Here's how the part is built. I have some questions about the finished solid (model axes, mm). A direction names the side the tool comes from. Round coordinates to 2 decimals unless told otherwise and drop trailing zeros. Order: outer loops, then holes, each group sorted by start corner. A loop starts at its lowest first (then second) coordinate and runs counter-clockwise, first axis right, second up. Notation, with made-up numbers: (68, -35.75) -> (77, -35.75) arc R37 ccw to (77, 0.25) -> close; hole circle Ø9 at (52, 25.5). An arc over 180 degrees is marked (long way). Answer in a Markdown table with one row per item.
```python
from build123d import *

# Parameters (mm, degrees)
SKETCH2_W     = 0.9
SKETCH2_H     = 0.2
CHAMFER1_SIZE = 0.8
CHAMFER2_SIZE = 0.3


with BuildPart() as part:
    # Sketch1 → Revolve1 (revolve)
    with BuildSketch(Plane(origin=(0, 0, 0), x_dir=(0, 0, -1), z_dir=(1, 0, 0))):
        Polygon((-400, 0), (400, 0), (400, 4), (390, 4), (390, 6.32), (-346, 6.32), (-346, 4.94), (-385, 4.94), (-385, 4), (-400, 4), align=None)
    revolve(axis=Axis((0, 0, 400), (0, 0, -1)))

    # Sketch2 → Cut-Revolve1 (revolve, cut)
    with BuildSketch(Plane(origin=(0, 0, 0), x_dir=(0, 0, -1), z_dir=(1, 0, 0))):
        with Locations((397.45, 3.9)):
            Rectangle(SKETCH2_W, SKETCH2_H)
    revolve(axis=Axis((0, 0, -400), (0, 0, 1)), mode=Mode.SUBTRACT)

    # Chamfer1
    chamfer1_edges = [part.edges().sort_by_distance(p)[0] for p in [
        (0, -4, -400),
    ]]
    chamfer(chamfer1_edges, length=CHAMFER1_SIZE)

    # Chamfer2
    chamfer2_edges = [part.edges().sort_by_distance(p)[0] for p in [
        (0, -4.94, 385),
        (0, -4, 400),
    ]]
    chamfer(chamfer2_edges, length=CHAMFER2_SIZE)


solid = part.part
```
1. For faces 1 (the face through (-2, -5, 346)), 2 (the face through (-1.3, -4.1, -390)), 3 (the face through (5.329, 3.398, -16.848)), which set-ups out of +Z, -Z, +X, -X, +Y, -Y let a thin tool reach every point of the face, with its end or its side?
Numbers:
| item | result |
|---|---|
| face 1 | +Z |
| face 2 | -Z |
| face 3 | +Z, -Z |
2. For pin 1 Ø2 at (x, z) = (4.5, -181.5) entering from +Y; pin 2 Ø6 at (y, z) = (5, -158.5) entering from -X; pin 3 Ø1.5 at (x, y) = (2.5, 4.5) entering from +Z, each with a flat end and sliding along its axis, tell me the tip position at first contact or that it passes through.
Numbers:
| item | result |
|---|---|
| pin 1 | stops at y = 5.26 |
| pin 2 | stops at x = -6 |
| pin 3 | stops at z = 385 |
3. Please list where these lines run through material, in increasing order: line 1 along X through (y, z) = (4, -225.5); line 2 along X through (y, z) = (0.25, -37); line 3 along Z through (x, y) = (0.25, 4.5).
Numbers:
| item | result |
|---|---|
| line 1 | x = -4.89 to 4.89 |
| line 2 | x = -6.32 to 6.32 |
| line 3 | z = -390 to 385 |
4. Suppose I cut it at C-C on z = -184.5. Write out the boundary of the cut face in (x, y), then the cut area to 3 significant figures.
Numbers:
| item | result |
|---|---|
| outline | circle Ø12.64 at (0, 0) |
| area | 125 mm2 |
